Job drawing, mm, ordinate dimensions from the low corner. One solid piece. Round coordinates to 2 decimals unless told otherwise and drop trailing zeros. Loops run counter-clockwise (first coordinate to the right, second up) from the corner with the lowest first, then second, coordinate; pieces in that order, holes last.
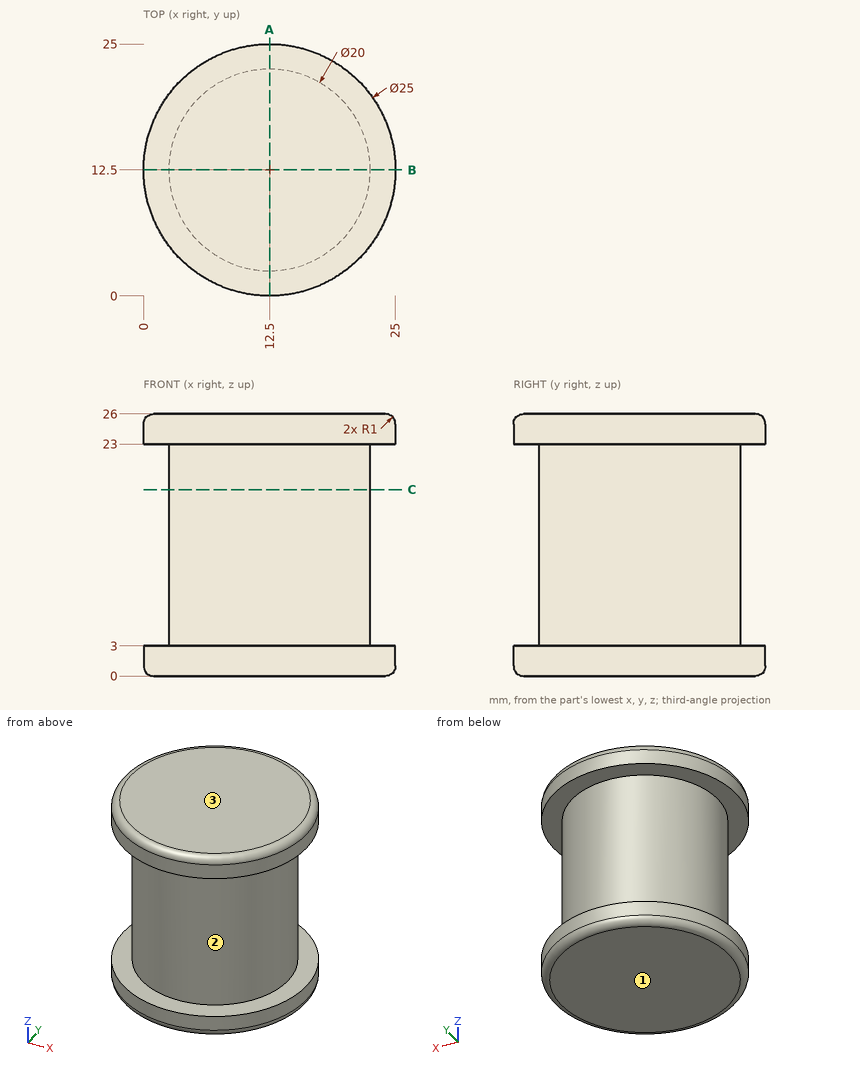
1) Slice it at A-A, the plane x = 12.5. Give the cut face in (y, z), then the cut area to 3 significant figures.
Values:
outline: (0, 1) arc R1 ccw to (1, 0) - (24, 0) arc R1 ccw to (25, 1) - (25, 3) - (22.5, 3) - (22.5, 23) - (25, 23) - (25, 25) arc R1 ccw to (24, 26) - (1, 26) arc R1 ccw to (0, 25) - (0, 23) - (2.5, 23) - (2.5, 3) - (0, 3) - close
area: 549 mm2
2) Wall check: line 1 along Z through (x, y) = (7.5, 21.5); line 2 along Z through (x, y) = (21.75, 20); line 3 along Y through (x, z) = (4.25, 9). Give the ranges that are in metal, low to high.
Values:
line 1: z = 0 to 3, 23 to 26
line 2: z = 0.09 to 3, 23 to 25.91
line 3: y = 6.85 to 18.15
3) Drop flat-ended pins along their axis: pin 1 Ø8 at (x, z) = (3, 21.5) entering from +Y; pin 2 Ø3 at (y, z) = (17.5, 20) entering from +X; pin 3 Ø6 at (x, z) = (15.5, 13.5) entering from +Y. Give the stop position or say it passes through.
Values:
pin 1: stops at y = 23.58
pin 2: stops at x = 21.87
pin 3: stops at y = 22.5
4) Mould opens along Z. For the marked faces 1, 2 and 3 say: released by +Z, released by -Z, zero draft, split by the parting line, or undercut.
Values:
face 1: released by -Z
face 2: undercut
face 3: released by +Z
5) Slice it at C-C, the plane z = 18.5. Give the cut face in (x, y), then the cut area to 3 significant figures.
Values:
outline: circle Ø20 at (12.5, 12.5)
area: 314 mm2
